```python
from build123d import *

# Parameters (mm, degrees)
SKETCH1_R           = 4
SKETCH1_R_2         = 1.5
BOSS_EXTRUDE1_DEPTH = 4
SKETCH2_OUTSIDE_W   = 12.4
SKETCH2_OUTSIDE_H   = 12.4
SKETCH2_OUTSIDE_R   = 2.75
CUT_EXTRUDE1_DEPTH  = 1.5
CHAMFER1_SIZE       = 1.25


with BuildPart() as part:
    # Sketch1 → Boss-Extrude1 (new body)
    with BuildSketch(Plane(origin=(0, 0, 0), x_dir=(0, 0, -1), z_dir=(1, 0, 0))):
        Circle(SKETCH1_R)
        Circle(SKETCH1_R_2, mode=Mode.SUBTRACT)
    extrude(amount=BOSS_EXTRUDE1_DEPTH)

    # Sketch2 outside → Cut-Extrude1 (cut)
    with BuildSketch(Plane(origin=(4, 0, 0), x_dir=(0, 0, -1), z_dir=(1, 0, 0))):
        Rectangle(SKETCH2_OUTSIDE_W, SKETCH2_OUTSIDE_H)
        Circle(SKETCH2_OUTSIDE_R, mode=Mode.SUBTRACT)
    extrude(amount=-CUT_EXTRUDE1_DEPTH, mode=Mode.SUBTRACT)

    # Chamfer1
    chamfer1_edges = [part.edges().sort_by_distance(p)[0] for p in [
        (2.5, 0, 4),
    ]]
    chamfer(chamfer1_edges, length=CHAMFER1_SIZE - 0.0001)  # a hair under: the kernel refuses the full size


solid = part.part
```
The listing builds one solid part. Answer for the finished solid, in the listing's coordinates (mm). Give positions to 0.01 mm unless a question says otherwise; leave off trailing zeros. Loops run counter-clockwise (first coordinate to the right, second up) from the corner with the lowest first, then second, coordinate; pieces in that order, holes last. Notation, with made-up numbers: M 44,69 L 52,69 A19 ccw 52,79 Z; hole C -30,-28.5 d6. An arc over 180 degrees is marked long. One line per item, written item: value.
Q1. A cutting plane is placed at C-C on x = 0.6. Determine the outline of the cut face in (y, z), then the cut area to 3 significant figures.
Working result:
outline: C 0,0 d8; hole C 0,0 d3
area: 43.2 mm^2
Q2. Determine the mould class of faces 1 (the face through (3.26, -2.685, 0.596)), 2 (the face through (1.97, 0.07, 1.5)), 3 (the face through (4, -1.2, -1.2)) for opening direction Y: +Y half, -Y half, draft (parallel to the pull), parting line (faces both ways), or undercut.
Working result:
face 1: parting line
face 2: undercut
face 3: draft
Q3. A cutting plane is placed at D-D on x = 1.5. Determine the outline of the cut face in (y, z), then the cut area to 3 significant figures.
Working result:
outline: C 0,0 d7.5; hole C 0,0 d3
area: 37.1 mm^2
Q4. Flat-ended cylindrical pins translate along their axes: P1, Ø1, axis at x = 1, z = -2.5, coming from the -Y side; P2, Ø1, axis at x = 1.5, y = -1.5, coming from the -Z side. Find the tip coordinate at first contact, or state that the pin passes through.
Working result:
P1: stops at y = -3.46
P2: stops at z = -3.86
Q5. Find the intervals of material crossed by line 1 (Y direction, x = 3.1, z = 0); line 2 (Y direction, x = 1.05, z = 0); line 3 (Z direction, x = 2.8, y = -1.25), in increasing order. Write a range as from..to.
Working result:
line 1: y = -2.75..-1.5, 1.5..2.75
line 2: y = -4..-1.5, 1.5..4
line 3: z = -2.45..-0.83, 0.83..2.45
